Check sheet for the modelled part. Datum: model origin and axes. Units: mm. A direction names the side the tool comes from. Round coordinates to 2 decimals unless told otherwise and drop trailing zeros. Order: outer loops, then holes, each group sorted by start corner. A loop starts at its lowest first (then second) coordinate and runs counter-clockwise, first axis right, second up. Notation, with made-up numbers: M 56.25,48.25 L 95.25,48.25 A24 cw 95.25,77.25 Z; hole C 68.5,31.25 d11. An arc over 180 degrees is marked long. One line per item, written item: value. Start each with the question number.
(1) Thickness scan on L1, parallel to Z at x = 9.5, y = 3.75; L2, parallel to X at y = 21, z = -20.5; L3, parallel to Z at x = 30, y = 17.5. Record the ranges inside material, lowest first.
(2) Cross-section at A-A, the plane x = 0. Enter the section's corners in (y, z) (3 decimals).
(3) Access from +Z, -Z, +X, -X, +Y, -Y to the whole of each face (thin tool, end or side, straight path). Record for faces 4 (the face through (30.873, 17.395, 2.617)), 5 (the face through (15.02, 9.96, -47.69)), 6 (the face through (-21, 25, 21)).
(4) Release check for a two-part mould opening along Z. For faces 1 (the face through (-49.529, 7.156, 10.998)), 2 (the face through (-0.092, 12.325, -30.984)), 3 (the face through (-46, 20, -9)) record: released by +Z, released by -Z, zero draft, split by the parting line, or undercut.
(5) Depth check by flat-ended pin: pin 1 Ø2 at (x, y) = (-15.5, 19.5) entering from +Z; pin 2 Ø3 at (y, z) = (15, 10) entering from +X; pin 3 Ø1.5 at (y, z) = (21.5, 25) entering from +X. Enter the tip coordinate at first touch or a pass-through.
Autodesk Inventor part; units mm, degrees
ref_plane "YZ Plane" through (0, 0, 0) normal (1, 0, 0) x (0, 1, 0)
ref_plane "XZ Plane" through (0, 0, 0) normal (0, 1, 0) x (-1, 0, 0)
ref_plane "XY Plane" through (0, 0, 0) normal (0, 0, 1) x (1, 0, 0)
sketch "Sketch1" plane through (0, 0, 0) normal (1, 0, 0) x (0, 1, 0)
  line L0 (25, -28.535) -> (25, -46)
  line L1 (25, -46) -> (20, -46)
  line L2 (20, -46) -> (20, -61.75)
  line L3 (20, -61.75) -> (18, -61.75)
  line L4 (18, -61.75) -> (12.5, -50)
  line L5 (12.5, -50) -> (7.5, -50)
  line L6 (2, -61.75) -> (0, -61.75)
  line L7 (7.5, -50) -> (2, -61.75)
  line L8 (-5, 0) -> (30, 0)
  line L9 (0, -61.75) -> (0, -26.985)
  line L10 (25, -28.535) -> (0, -26.985)
  point P0 (0, 0)
  point P1 (10, -50)
  dimension "d4" = 5
  dimension "d5" = 2
  dimension "d24" = 28.535
  dimension "d26" = 5
  dimension "d27" = 17.465
  dimension "d29" = 26.985
  dimension "d30" = 61.75
  dimension "d31" = 25
  dimension "d32" = 50
revolve "Revolution1" add sketch "Sketch1" angle 360 about axis through (0, -10, 0) along (0, 1, 0)
fillet "Fillet1" radius 1 1 edges at (0, 25, 46)
fillet "Fillet2" radius 0.5 2 edges at (0, 20, 61.75) (0, 0, 61.75)
sketch "Sketch5" plane through (0, 25, 0) normal (0, 1, 0) x (1, 0, 0)
  circle A0 centre (0, 0) radius 26.985
  line L0 (0, 0) -> (0, 26.985) construction
hole "Hole1" at (0, 25, -26.985) direction (0, -1, 0) diameter 8 end through all
sketch "Sketch6" plane through (0, 25, 0) normal (0, 1, 0) x (1, 0, 0)
  line L0 (0, 0) -> (26.8823, -2.3519) construction
  arc A0 (-3.989, 26.6885) -> (3.989, 26.6885) centre (0, 0) ccw
  line L1 (0, 0) -> (0, -26.985) construction
  line L2 (0, 0) -> (-26.8823, -2.3519) construction
  dimension "d40" = 85
  dimension "d41" = 85
hole "Hole2" at (26.8823, 25, 2.3519) at (-26.8823, 25, 2.3519) direction (0, -1, 0) diameter 8 depth 15 tip angle 118
equation "\"d41\" = d40"
properties part number "Шкив 118 мм"
Values found:
1. L1: -57.23 to -25.51, 25.51 to 57.23
1. L2: -41.18 to -19.49, 19.49 to 41.18
1. L3: -52.75 to -0.15, 4.86 to 52.75
2. outline: M 0,-61.25 A0.5 ccw 0.5,-61.75 L 2,-61.75 L 7.5,-50 L 12.5,-50 L 18,-61.75 L 19.5,-61.75 A0.5 ccw 20,-61.25 L 20,-46 L 24,-46 A1 ccw 25,-45 L 25,-30.985 L 0,-30.985 Z; M 0,26.985 L 25,28.535 L 25,45 A1 ccw 24,46 L 20,46 L 20,61.25 A0.5 ccw 19.5,61.75 L 18,61.75 L 12.5,50 L 7.5,50 L 2,61.75 L 0.5,61.75 A0.5 ccw 0,61.25 Z
3. face 4: +Y
3. face 5: none
3. face 6: +Z, -Z, +X, -X, +Y
4. face 1: split by the parting line
4. face 2: undercut
4. face 3: zero draft
5. pin 1: z = 60.02
5. pin 2: x = 57.7
5. pin 3: x = 39.09
